Can you work these out from the drawing? Everything is in mm from the part's minimum corner. Give positions to 0.01 mm unless a question says otherwise; leave off trailing zeros. Write each loop counter-clockwise with the first axis right and the second up, starting at its lowest first coordinate (ties: lowest second). Pieces come first, ordered by that corner, then holes. Notation, with made-up numbers: (1, 46) - (8, 46) arc R5 ccw to (8, 50) - close; hole circle Ø5 at (-29.75, 16). An arc over 180 degrees is marked (long way). Use a Markdown table: item, result.
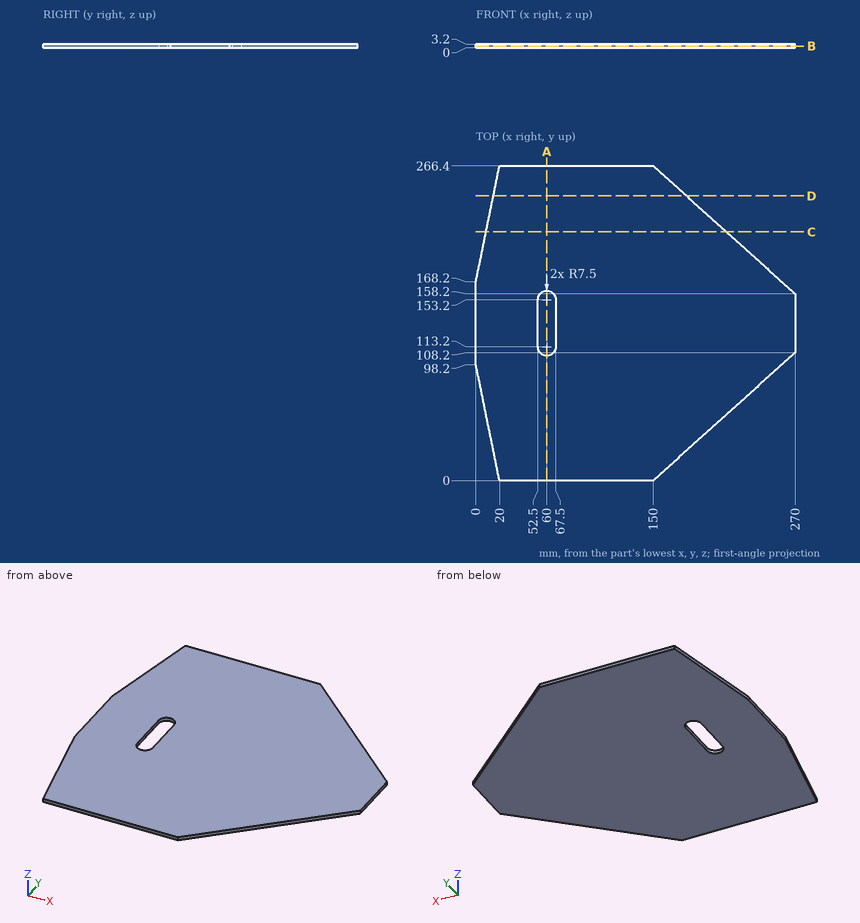
Item 1: I need wall thicknesses on line 1 along X through (y, z) = (127, 3.05); line 2 along X through (y, z) = (107, 0.2); line 3 along Y through (x, z) = (65, 0.6). Which ranges of each line are inside material? Lowest first, please. Write a range as [from, to].
Values:
| item | result |
|---|---|
| line 1 | x = [0, 52.5], [67.5, 270] |
| line 2 | x = [0, 55.78], [64.22, 268.67] |
| line 3 | y = [0, 107.61], [158.79, 266.4] |
Item 2: If we section it at A-A, the plane x = 60: Write out the boundary of the cut face in (y, z).
Values:
| item | result |
|---|---|
| outline | (0, 0) - (105.7, 0) - (105.7, 3.2) - (0, 3.2) - close; (160.7, 0) - (266.4, 0) - (266.4, 3.2) - (160.7, 3.2) - close |
Item 3: Will these pins go through, and if not, where does the flat tip stop? pin 1 Ø1.5 at (y, z) = (100, 2) entering from +X; pin 2 Ø1.5 at (x, z) = (241, 1.5) entering from +Y.
Values:
| item | result |
|---|---|
| pin 1 | stops at x = 261.74 |
| pin 2 | stops at y = 185.02 |
Item 4: If we section it at D-D, the plane y = 241: Write out the boundary of the cut face in (x, z), plus the area to 3 significant figures.
Values:
| item | result |
|---|---|
| outline | (14.83, 0) - (178.17, 0) - (178.17, 3.2) - (14.83, 3.2) - close |
| area | 523 mm2 |
Item 5: If we section it at B-B, the plane z = 1.5: Write out the boundary of the cut face in (x, y), plus the area to 3 significant figures.
Values:
| item | result |
|---|---|
| outline | (0, 98.2) - (20, 0) - (150, 0) - (270, 108.2) - (270, 158.2) - (150, 266.4) - (20, 266.4) - (0, 168.2) - close; hole (52.5, 113.2) arc R7.5 ccw to (67.5, 113.2) - (67.5, 153.2) arc R7.5 ccw to (52.5, 153.2) - close |
| area | 56,200 mm2 |
Item 6: If we section it at C-C, the plane y = 210.5: Write out the boundary of the cut face in (x, z), plus the area to 3 significant figures.
Values:
| item | result |
|---|---|
| outline | (8.62, 0) - (212, 0) - (212, 3.2) - (8.62, 3.2) - close |
| area | 651 mm2 |
